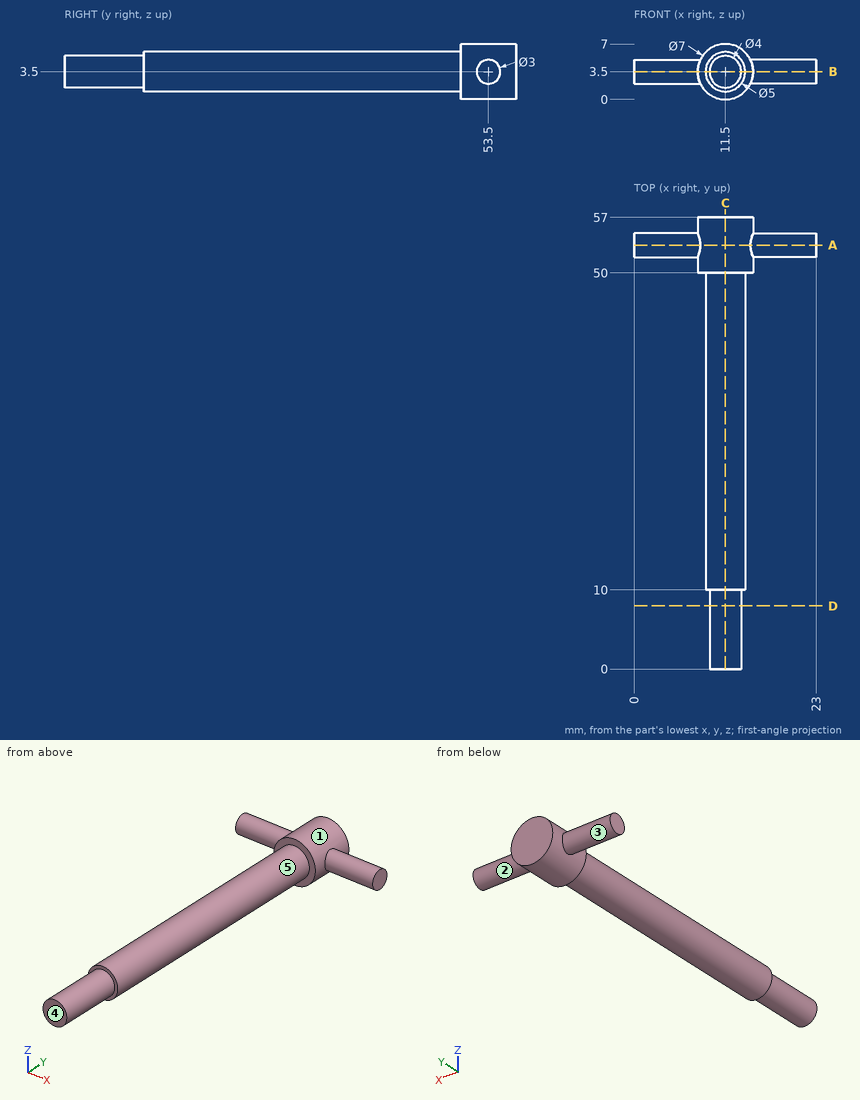
The drawing under review shows one solid part. Ordinate dimensions are in mm from its lowest x, y, z. A direction names the side the tool comes from. Coordinates: 2 decimals unless noted, no trailing zeros. Loops run counter-clockwise (first coordinate to the right, second up) from the corner with the lowest first, then second, coordinate; pieces in that order, holes last. Notation, with made-up numbers: (58.5, 10) - (75.5, 10) arc R26 cw to (75.5, 39) - close; hole circle Ø7 at (12, 48). An arc over 180 degrees is marked (long way). Use CSV: the item, a comma, the result in double quotes. Start each with the question number.
1. To check wall thickness, follow probe 1 along X at (y, z) = (22, 3.25); probe 2 along Y at (x, z) = (11, 6.25); probe 3 along Y at (x, z) = (17.75, 3.25). State the ranges of each line that lie inside material, in increasing order.
2. Add section D-D on y = 8. Give the boundary of the cut face in (x, z), plus the area to 3 significant figures.
3. Add section A-A on y = 53.5. Give the boundary of the cut face in (x, z).
4. For the marked faces 1, 2, 3, 4 and 5, list the 3-axis set-ups (+Z, -Z, +X, -X, +Y, -Y) from which the entire face can be reached by the end or side of a thin tool; tool diameter is ignored.
5. Add section B-B on z = 3.5. Give the boundary of the cut face in (x, y), plus the area to 3 significant figures.
6. Clearance check with flat-ended pins moving along their axes: pin 1 (1.5 mm diameter, centred on y = 31.5, z = 6, fed in from +X); pin 2 (4 mm diameter, centred on x = 19, z = 4.5, fed in from +Y); pin 3 (5 mm diameter, centred on x = 7, y = 28, fed in from -Z). State where each tip first meets the part, or that it passes through.
7. Add section C-C on x = 11.5. Give the boundary of the cut face in (y, z), plus the area to 3 significant figures.
Resolved:
1,probe 1,"9.01 to 13.99"
1,probe 2,"50 to 57"
1,probe 3,"52.02 to 54.98"
2,outline,"circle Ø4 at (11.5, 3.5)"
2,area,"12.6 mm2"
3,outline,"(0, 2) - (8.34, 2) arc R3.5 ccw to (14.66, 2) - (23, 2) - (23, 5) - (14.66, 5) arc R3.5 ccw to (8.34, 5) - (0, 5) - close"
4,face 1,"none"
4,face 2,"+X"
4,face 3,"-X"
4,face 4,"+Z, -Z, +X, -X, -Y"
4,face 5,"-Y"
5,outline,"(0, 52) - (8, 52) - (8, 50) - (9, 50) - (9, 10) - (9.5, 10) - (9.5, 0) - (13.5, 0) - (13.5, 10) - (14, 10) - (14, 50) - (15, 50) - (15, 52) - (23, 52) - (23, 55) - (15, 55) - (15, 57) - (8, 57) - (8, 55) - (0, 55) - close"
5,area,"337 mm2"
6,pin 1,"x = 13.29"
6,pin 2,"y = 55"
6,pin 3,"z = 2"
7,outline,"(0, 1.5) - (10, 1.5) - (10, 1) - (50, 1) - (50, 0) - (57, 0) - (57, 7) - (50, 7) - (50, 6) - (10, 6) - (10, 5.5) - (0, 5.5) - close"
7,area,"289 mm2"
